from build123d import *

# Parameters (mm, degrees)
EXTRUDE_1_DEPTH     = 3
CUT_EXTRUDE_START   = -10
CUT_EXTRUDE_1_DEPTH = 10
SKETCH_3_W          = 20
SKETCH_3_H          = 40
EXTRUDE_2_DEPTH     = 3
FILLET_2_R          = 1
FILLET_3_R          = 1
SKETCH_5_R          = 1.5
CUT_EXTRUDE_2_DEPTH = 10
SKETCH_6_R          = 1.5
CUT_EXTRUDE_3_DEPTH = 10
SKETCH_8_R          = 1.5
CUT_EXTRUDE_4_DEPTH = 234.216551728
SKETCH_10_R         = 4
CUT_EXTRUDE_6_DEPTH = 234.216551728
SKETCH_11_W         = 40.88
SKETCH_11_H         = 149.99999794
CUT_EXTRUDE_7_DEPTH = 10
SKETCH_12_W         = 75.865569995
SKETCH_12_H         = 55.877442545
CUT_EXTRUDE_8_DEPTH = 10


with BuildPart() as part:
    # 草图1 → 凸台-拉伸1 (new body)
    with BuildSketch(Plane(origin=(0, 0, 0), x_dir=(1, 0, 0), z_dir=(0, 1, 0))):
        with BuildLine():
            Line((-130, -193.6), (-50, -193.6))
            Line((-50, -193.6), (50, -193.6))
            Line((50, -193.6), (130, -193.6))
            Line((130, -193.6), (130, -173.6))
            Line((130, -173.6), (60, -173.6))
            ThreePointArc((60, -173.6), (52.928932188, -170.671067812), (50, -163.6))
            Line((50, -163.6), (50, -105))
            ThreePointArc((50, -105), (52.928932188, -97.928932188), (60, -95))
            Line((60, -95), (130, -95))
            Line((130, -95), (130, -75))
            Line((130, -75), (130, 75))
            Line((130, 75), (130, 95))
            Line((130, 95), (60, 95))
            ThreePointArc((60, 95), (52.928932188, 97.928932188), (50, 105))
            Line((50, 105), (50, 163.6))
            ThreePointArc((50, 163.6), (52.928932188, 170.671067812), (60, 173.6))
            Line((60, 173.6), (130, 173.6))
            Line((130, 173.6), (130, 193.6))
            Line((130, 193.6), (50, 193.6))
            Line((50, 193.6), (-50, 193.6))
            Line((-50, 193.6), (-130, 193.6))
            Line((-130, 193.6), (-130, 173.6))
            Line((-130, 173.6), (-60, 173.6))
            ThreePointArc((-60, 173.6), (-52.928932188, 170.671067812), (-50, 163.6))
            Line((-50, 163.6), (-50, 105))
            ThreePointArc((-50, 105), (-52.928932188, 97.928932188), (-60, 95))
            Line((-60, 95), (-130, 95))
            Line((-130, 95), (-130, 75))
            Line((-130, 75), (-130, -75))
            Line((-130, -75), (-130, -95))
            Line((-130, -95), (-60, -95))
            ThreePointArc((-60, -95), (-52.928932188, -97.928932188), (-50, -105))
            Line((-50, -105), (-50, -163.6))
            ThreePointArc((-50, -163.6), (-52.928932188, -170.671067812), (-60, -173.6))
            Line((-60, -173.6), (-130, -173.6))
            Line((-130, -173.6), (-130, -193.6))
        make_face()
    extrude(amount=EXTRUDE_1_DEPTH)

    # 草图2 → 切除-拉伸1 (cut)
    with BuildSketch(Plane(origin=(0, 3, 0), x_dir=(1, 0, 0), z_dir=(0, 1, 0)).offset(CUT_EXTRUDE_START)):
        with BuildLine():
            Line((-130, 95), (-130, -75))
            Line((-130, -75), (130, -75))
            Line((130, -75), (130, 95))
            Line((130, 95), (60, 95))
            ThreePointArc((60, 95), (52.928932188, 97.928932188), (50, 105))
            Line((50, 105), (50, 163.6))
            ThreePointArc((50, 163.6), (52.928932188, 170.671067812), (60, 173.6))
            Line((60, 173.6), (130, 173.6))
            Line((130, 173.6), (130, 193.6))
            Line((130, 193.6), (-130, 193.6))
            Line((-130, 193.6), (-130, 173.6))
            Line((-130, 173.6), (-60, 173.6))
            ThreePointArc((-60, 173.6), (-52.928932188, 170.671067812), (-50, 163.6))
            Line((-50, 163.6), (-50, 105))
            ThreePointArc((-50, 105), (-52.928932188, 97.928932188), (-60, 95))
            Line((-60, 95), (-130, 95))
        make_face()
    extrude(amount=CUT_EXTRUDE_1_DEPTH, mode=Mode.SUBTRACT)

    # 草图3 → 凸台-拉伸2 (add)
    with BuildSketch(Plane(origin=(0, 3, 0), x_dir=(1, 0, 0), z_dir=(0, 1, 0))):
        with Locations((90, -55)):
            Rectangle(SKETCH_3_W, SKETCH_3_H)
        with Locations((-90, -55)):
            Rectangle(SKETCH_3_W, SKETCH_3_H)
    extrude(amount=-EXTRUDE_2_DEPTH)

    # 圆角2
    fillet_2_edges = [part.edges().sort_by_distance(p)[0] for p in [
        (-130, 1.5, 75),
        (-100, 1.5, 35),
        (-80, 1.5, 35),
        (-130, 1.5, 193.6),
        (-130, 1.5, 173.6),
        (-130, 1.5, 95),
    ]]
    fillet(fillet_2_edges, radius=FILLET_2_R)

    # 圆角3
    fillet_3_edges = [part.edges().sort_by_distance(p)[0] for p in [
        (130, 1.5, 75),
        (80, 1.5, 35),
        (100, 1.5, 35),
        (130, 1.5, 95),
        (130, 1.5, 173.6),
        (130, 1.5, 193.6),
    ]]
    fillet(fillet_3_edges, radius=FILLET_3_R)

    # 草图5 → 切除-拉伸2 (cut)
    with BuildSketch(Plane(origin=(0, 3, 0), x_dir=(1, 0, 0), z_dir=(0, 1, 0))):
        with Locations(Location((22, -112.3, 0), (0, 0, 270))):
            Circle(SKETCH_5_R)
        with Locations(Location((-22, -112.3, 0), (0, 0, 270))):
            Circle(SKETCH_5_R)
        with Locations(Location((-22, -156.3, 0), (0, 0, 270))):
            Circle(SKETCH_5_R)
        with Locations(Location((22, -156.3, 0), (0, 0, 270))):
            Circle(SKETCH_5_R)
    extrude(amount=-CUT_EXTRUDE_2_DEPTH, mode=Mode.SUBTRACT)

    # 草图6 → 切除-拉伸3 (cut)
    with BuildSketch(Plane(origin=(0, 3, 0), x_dir=(1, 0, 0), z_dir=(0, 1, 0))):
        with Locations(Location((120, -85, 0), (0, 0, 270))):
            Circle(SKETCH_6_R)
        with Locations(Location((80, -85, 0), (0, 0, 270))):
            Circle(SKETCH_6_R)
        with Locations(Location((100, -85, 0), (0, 0, 270))):
            Circle(SKETCH_6_R)
        with Locations(Location((60, -85, 0), (0, 0, 270))):
            Circle(SKETCH_6_R)
        with Locations(Location((40, -85, 0), (0, 0, 270))):
            Circle(SKETCH_6_R)
        with Locations(Location((20, -85, 0), (0, 0, 270))):
            Circle(SKETCH_6_R)
        with Locations(Location((0, -85, 0), (0, 0, 270))):
            Circle(SKETCH_6_R)
        with Locations(Location((-20, -85, 0), (0, 0, 270))):
            Circle(SKETCH_6_R)
        with Locations(Location((-40, -85, 0), (0, 0, 270))):
            Circle(SKETCH_6_R)
        with Locations(Location((-60, -85, 0), (0, 0, 270))):
            Circle(SKETCH_6_R)
        with Locations(Location((-80, -85, 0), (0, 0, 270))):
            Circle(SKETCH_6_R)
        with Locations(Location((-100, -85, 0), (0, 0, 270))):
            Circle(SKETCH_6_R)
        with Locations(Location((-120, -85, 0), (0, 0, 270))):
            Circle(SKETCH_6_R)
        with Locations(Location((-100, -183.6, 0), (0, 0, 270))):
            Circle(SKETCH_6_R)
        with Locations(Location((-120, -183.6, 0), (0, 0, 270))):
            Circle(SKETCH_6_R)
        with Locations(Location((-80, -183.6, 0), (0, 0, 270))):
            Circle(SKETCH_6_R)
        with Locations(Location((-60, -183.6, 0), (0, 0, 270))):
            Circle(SKETCH_6_R)
        with Locations(Location((-40, -183.6, 0), (0, 0, 270))):
            Circle(SKETCH_6_R)
        with Locations(Location((-20, -183.6, 0), (0, 0, 270))):
            Circle(SKETCH_6_R)
        with Locations(Location((0, -183.6, 0), (0, 0, 270))):
            Circle(SKETCH_6_R)
        with Locations(Location((20, -183.6, 0), (0, 0, 270))):
            Circle(SKETCH_6_R)
        with Locations(Location((40, -183.6, 0), (0, 0, 270))):
            Circle(SKETCH_6_R)
        with Locations(Location((60, -183.6, 0), (0, 0, 270))):
            Circle(SKETCH_6_R)
        with Locations(Location((80, -183.6, 0), (0, 0, 270))):
            Circle(SKETCH_6_R)
        with Locations(Location((100, -183.6, 0), (0, 0, 270))):
            Circle(SKETCH_6_R)
        with Locations(Location((120, -183.6, 0), (0, 0, 270))):
            Circle(SKETCH_6_R)
    extrude(amount=-CUT_EXTRUDE_3_DEPTH, mode=Mode.SUBTRACT)

    # 草图8 → 切除-拉伸4 (cut, through all)
    with BuildSketch(Plane.XZ):
        with Locations(Location((-90, 40, 0), (0, 0, 270))):
            Circle(SKETCH_8_R)
        with Locations(Location((-90, 60, 0), (0, 0, 270))):
            Circle(SKETCH_8_R)
        with Locations(Location((90, 60, 0), (0, 0, 270))):
            Circle(SKETCH_8_R)
        with Locations(Location((90, 40, 0), (0, 0, 270))):
            Circle(SKETCH_8_R)
    extrude(amount=-CUT_EXTRUDE_4_DEPTH, mode=Mode.SUBTRACT)

    # 草图10 → 切除-拉伸6 (cut, through all)
    with BuildSketch(Plane(origin=(0, 3, 0), x_dir=(1, 0, 0), z_dir=(0, 1, 0))):
        with Locations((-100, -75)):
            Circle(SKETCH_10_R)
        with Locations((-80, -75)):
            Circle(SKETCH_10_R)
        with Locations((80, -75)):
            Circle(SKETCH_10_R)
        with Locations((100, -75)):
            Circle(SKETCH_10_R)
    extrude(amount=-CUT_EXTRUDE_6_DEPTH, mode=Mode.SUBTRACT)

    # 草图11 → 切除-拉伸7 (cut)
    with BuildSketch(Plane(origin=(0, 3, 0), x_dir=(1, 0, 0), z_dir=(0, 1, 0))):
        with Locations((-98.325151621, -1.03e-06)):
            Rectangle(SKETCH_11_W, SKETCH_11_H)
    extrude(amount=-CUT_EXTRUDE_7_DEPTH, mode=Mode.SUBTRACT)

    # 草图12 → 切除-拉伸8 (cut)
    with BuildSketch(Plane(origin=(0, 3, 0), x_dir=(1, 0, 0), z_dir=(0, 1, 0))):
        with Locations((78.567215003, -47.061278728)):
            Rectangle(SKETCH_12_W, SKETCH_12_H)
    extrude(amount=-CUT_EXTRUDE_8_DEPTH, mode=Mode.SUBTRACT)


solid = part.part
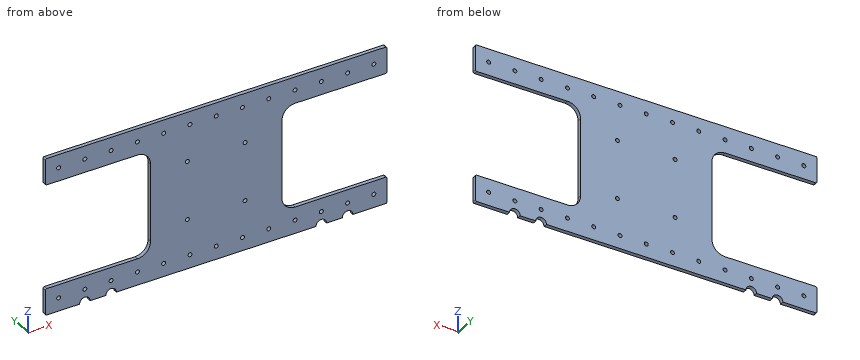
The listing builds one solid part. Answer for the finished solid, in the listing's coordinates (mm). Round coordinates to 2 decimals unless told otherwise and drop trailing zeros. Loops run counter-clockwise (first coordinate to the right, second up) from the corner with the lowest first, then second, coordinate; pieces in that order, holes last. Notation, with made-up numbers: M -34.75,3 L -1.75,3 A14 ccw -1.75,22 Z; hole C -35.5,69.25 d1. An arc over 180 degrees is marked long. Write each question's results on one line, items separated by ' | '. Start each with the question number.
1) Each of these flat-tipped pins is pushed along its axis until it touches: pin 1 (5 mm diameter, centred on x = -40, z = 85, fed in from -Y); pin 2 (1 mm diameter, centred on y = 2.5, z = 112.5, fed in from -X); pin 3 (1.8 mm diameter, centred on x = 80, z = 183.6, fed in from -Y). Where does it stop, or does it pass through?
2) Find section B-B on z = 145.5. Write down the section's boundary in (x, y), plus the area to 3 significant figures.
3) Straight lines are drawn through the part: probe 1 along Z at (x, y) = (100, 1.65); probe 2 along X at (y, z) = (1.3, 156.5); probe 3 along Z at (x, y) = (-120, 2.2). For each, find the intervals that lie inside material, in ascending order.
4) Find section A-A on x = 92.5. Write down the section's boundary in (y, z).
5) Find section C-C on y = 2.5. Count the separate pieces of the cut face and the enclosed holes in it, plus the area to 3 significant figures.
Final values:
1) pin 1: y = 0 | pin 2: x = -50 | pin 3: through
2) outline: M -50,0 L 50,0 L 50,3 L -50,3 Z | area: 300 mm²
3) probe 1: 79 to 83.5, 86.5 to 95, 173.6 to 182.1, 185.1 to 193.6 | probe 2: -50 to -23.49, -20.51 to 20.51, 23.49 to 50 | probe 3: 75 to 83.5, 86.5 to 95, 173.6 to 182.1, 185.1 to 193.6
4) outline: M 0,75 L 3,75 L 3,95 L 0,95 Z; M 0,173.6 L 3,173.6 L 3,193.6 L 0,193.6 Z
5) separate pieces: 1 | enclosed holes: 30 | area: 18,000 mm²
